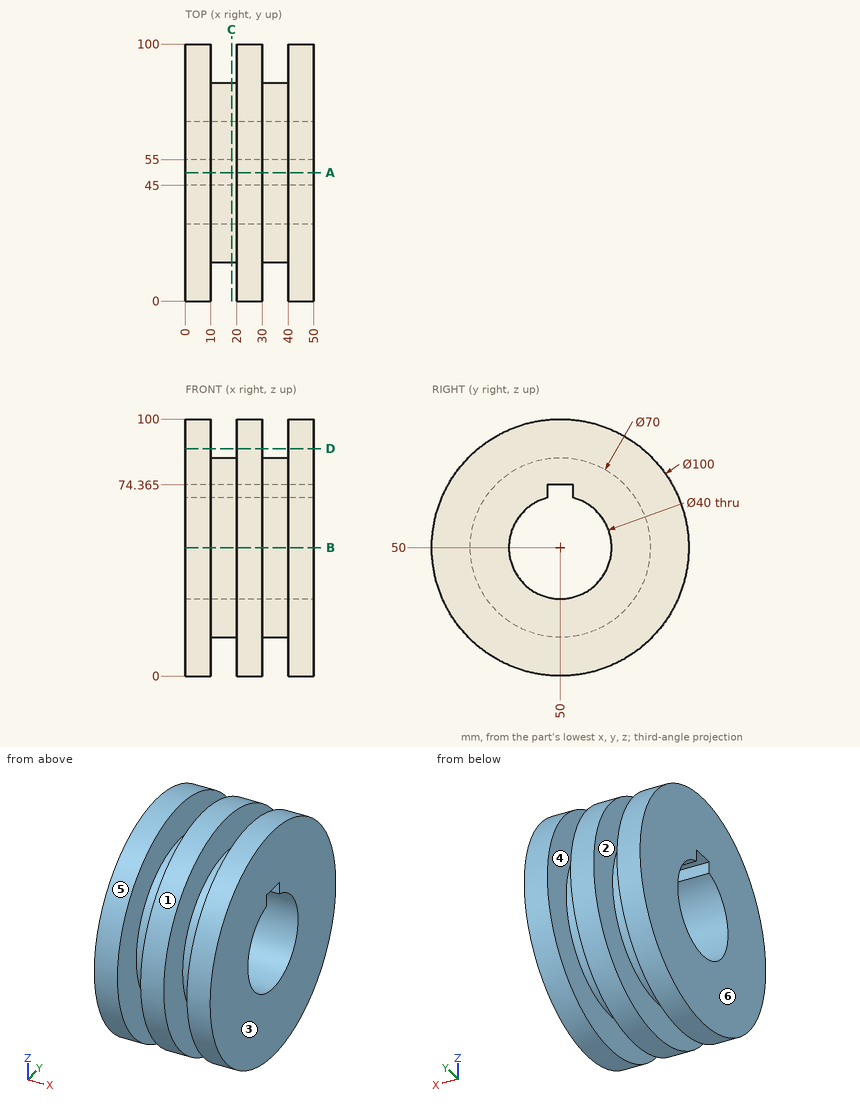
Job drawing, mm, ordinate dimensions from the low corner. One solid piece. A direction names the side the tool comes from. Round coordinates to 2 decimals unless told otherwise and drop trailing zeros. Loops run counter-clockwise (first coordinate to the right, second up) from the corner with the lowest first, then second, coordinate; pieces in that order, holes last.
(1) Cut at D-D (z = 88.5). Give the cut face in (x, y).
(2) Which spindle directions (+Z, -Z, +X, -X, +Y, -Y) get a long thin tool onto all of the face, cutting with end or side? Do the marked faces 1 and 2. Say none if no direction does.
(3) Two-plate mould, pull along X, no slides. Class the marked faces 3, 4, 5 and 6: +X half, -X half, draft (parallel to the pull), parting line (faces both ways), or undercut.
(4) Cut at B-B (z = 50). Give the cut face in (x, y), plus the area to 3 significant figures.
(5) Wall check: line 1 along X through (y, z) = (14, 71); line 2 along Z through (x, y) = (16.5, 50) (3 decimals); line 3 along Y through (x, z) = (45, 54). Give the ranges that are in metal, low to high.
(6) Cut at C-C (x = 18). Give the cut face in (y, z) (3 decimals), plus the area to 3 significant figures.
(7) Drop flat-ended pins along their axis: pin 1 (12 mm diameter, centred on x = 17, y = 59.5, fed in from -Z); pin 2 (8 mm diameter, centred on x = 28.5, y = 48.5, fed in from -Z); pin 3 (1.5 mm diameter, centred on x = 25.5, z = 10.5, fed in from -Y); pin 4 (1 mm diameter, centred on y = 84, z = 31.5, fed in from -X). Give the stop position or say it passes through.
(8) Cut at A-A (y = 50). Give the cut face in (x, z) (3 decimals).
Findings below:
1. outline: (0, 18.1) - (10, 18.1) - (10, 81.9) - (0, 81.9) - close; (20, 18.1) - (30, 18.1) - (30, 81.9) - (20, 81.9) - close; (40, 18.1) - (50, 18.1) - (50, 81.9) - (40, 81.9) - close
2. face 1: +X, -X
2. face 2: none
3. face 3: +X half
3. face 4: undercut
3. face 5: draft
3. face 6: -X half
4. outline: (0, 0) - (10, 0) - (10, 15) - (20, 15) - (20, 0) - (30, 0) - (30, 15) - (40, 15) - (40, 0) - (50, 0) - (50, 30) - (0, 30) - close; (0, 70) - (50, 70) - (50, 100) - (40, 100) - (40, 85) - (30, 85) - (30, 100) - (20, 100) - (20, 85) - (10, 85) - (10, 100) - (0, 100) - close
4. area: 2,400 mm2
5. line 1: x = 0 to 10, 20 to 30, 40 to 50
5. line 2: z = 15 to 30, 74.365 to 85
5. line 3: y = 0.16 to 30.4, 69.6 to 99.84
6. outline: circle Ø70 at (50, 50); hole (45, 69.365) arc R20 ccw (long way) to (55, 69.365) - (55, 74.365) - (45, 74.365) - close
6. area: 2,550 mm2
7. pin 1: stops at z = 0.19
7. pin 2: stops at z = 0
7. pin 3: stops at y = 18.4
7. pin 4: stops at x = 0
8. outline: (0, 0) - (10, 0) - (10, 15) - (20, 15) - (20, 0) - (30, 0) - (30, 15) - (40, 15) - (40, 0) - (50, 0) - (50, 30) - (0, 30) - close; (0, 74.365) - (50, 74.365) - (50, 100) - (40, 100) - (40, 85) - (30, 85) - (30, 100) - (20, 100) - (20, 85) - (10, 85) - (10, 100) - (0, 100) - close
